CAD build for the part. Positions are in the model's coordinates, mm. A direction names the side the tool comes from. Round coordinates to 2 decimals unless told otherwise and drop trailing zeros. Write each loop counter-clockwise with the first axis right and the second up, starting at its lowest first coordinate (ties: lowest second). Pieces come first, ordered by that corner, then holes. Notation, with made-up numbers: M -39.75,-6.5 L -31.75,-6.5 A26 cw -31.75,29.5 Z; hole C 15,23 d2. An arc over 180 degrees is marked long. Write each question's results on one line, items separated by ' | '. Start each with the question number.
```python
from build123d import *

# Parameters (mm, degrees)
ESQUISSE1_R                        = 11
BOSS_EXTRU_1_DEPTH                 = 5
ESQUISSE2_R                        = 1
ENL_V_MAT_EXTRU_1_DEPTH            = 6
ESQUISSE3_R                        = 5
BOSS_EXTRU_2_DEPTH                 = 57.75
BOSS_EXTRU_3_DEPTH                 = 15
CONG_1_R                           = 1
R_P_TITION_CIRCULAIRE1_COUNT       = 5
CONG_1_OF_R_P_TITION_CIRCULAIRE1_R = 1


with BuildPart() as part:
    # Esquisse1 → Boss.-Extru.1 (new body)
    with BuildSketch(Plane.XY):
        Circle(ESQUISSE1_R)
    extrude(amount=BOSS_EXTRU_1_DEPTH)

    # Esquisse2 → Enlèv. mat.-Extru.1 (cut, through all)
    with BuildSketch(Plane.XY.offset(5)):
        with Locations((0, 8)):
            Circle(ESQUISSE2_R)
        with Locations((0, -8)):
            Circle(ESQUISSE2_R)
    extrude(amount=-ENL_V_MAT_EXTRU_1_DEPTH, mode=Mode.SUBTRACT)

    # Esquisse3 → Boss.-Extru.2 (add)
    with BuildSketch(Plane.XY.offset(5)):
        Circle(ESQUISSE3_R)
    extrude(amount=BOSS_EXTRU_2_DEPTH)

    # Esquisse4 → Boss.-Extru.3 (add, symmetric)
    with BuildSketch(Plane.XY.offset(35)):
        with BuildLine():
            ThreePointArc((-2.731158071, 4.188170912), (-2.5, 7.120566641), (-1.5, 9.886859967))
            ThreePointArc((-1.5, 9.886859967), (0, 10), (1.5, 9.886859967))
            ThreePointArc((1.5, 9.886859967), (2.5, 7.120566641), (2.731158071, 4.188170912))
            ThreePointArc((2.731158071, 4.188170912), (0, -5), (-2.731158071, 4.188170912))
        make_face()
    boss_extru_3 = extrude(amount=BOSS_EXTRU_3_DEPTH, both=True)

    # Congé1
    cong_1_edges = [part.edges().sort_by_distance(p)[0] for p in [
        (1.5, 9.886859967, 35),
        (-1.5, 9.886859967, 35),
    ]]
    fillet(cong_1_edges, radius=CONG_1_R)

    # Répétition circulaire1: Boss.-Extru.3 ×5 about axis
    r_p_tition_circulaire1_axis = Axis((0, 0, 0), (0, 0, 1))
    for i in range(1, R_P_TITION_CIRCULAIRE1_COUNT):
        add(boss_extru_3.rotate(r_p_tition_circulaire1_axis, i * 360 / R_P_TITION_CIRCULAIRE1_COUNT))

    # Congé1 of Répétition circulaire1
    cong_1_of_r_p_tition_circulaire1_edges = [part.edges().sort_by_distance(p)[0] for p in [
        (-8.939437105, 4.481792525, 35),
        (-9.866488089, 1.628622976, 35),
        (-7.024875971, -7.116959856, 35),
        (-4.597824988, -8.880315612, 35),
        (4.597824988, -8.880315612, 35),
        (7.024875971, -7.116959856, 35),
        (9.866488089, 1.628622976, 35),
        (8.939437105, 4.481792525, 35),
    ]]
    fillet(cong_1_of_r_p_tition_circulaire1_edges, radius=CONG_1_OF_R_P_TITION_CIRCULAIRE1_R)


solid = part.part
```
1) Saw through at A-A, the plane y = 8. Write the cut outline in (x, z).
2) Drop flat-ended pins along their axis: pin 1 Ø4 at (y, z) = (0, 43.5) entering from +X; pin 2 Ø12 at (x, z) = (-7.5, 36) entering from -Y; pin 3 Ø5 at (x, z) = (-1.5, 42.5) entering from +Y; pin 4 Ø1.8 at (x, y) = (0, -8) entering from -Z. Give the stop position or say it passes through.
3) 3-axis set-ups, long thin cutter, end or side, ignore diameter. For faces 4 (the face through (9.507, 3.103, 35.21)), 5 (the face through (4.77, 1.5, 14.22)), 6 (the face through (4, -6, 50)), 7 (the face through (-1.927, -7.013, 35.21)), 8 (the face through (0, 9, 3)): which of +Z, -Z, +X, -X, +Y, -Y reach the whole face in a straight line?
4) Wall check: line 1 along Y through (x, z) = (0, 2.95); line 2 along Z through (x, y) = (4.5, -5.5); line 3 along X through (y, z) = (-0.25, 19.5). Give the ranges that are in metal, low to high. Write a range as from..to.
5) Pull direction X, two halves, no side cores. Call faces 1 (the face through (-7, 2, 50)), 2 (the face through (5.68, 4.54, 35.21)), 3 (the face through (6.074, -3.999, 35.21)): pulls with the +X half, pulls with the -X half, needs draft (parallel to the pull), parting line crosses it, or undercut.
6) Saw through at B-B, the plane z = 11. Write the cut outline in (x, y), plus the area to 3 significant figures.
Filled sheet:
1) outline: M -7.55,0 L -1,0 L -1,5 L -7.55,5 Z; M -2.27,20 L 2.27,20 L 2.27,50 L -2.27,50 Z; M 1,0 L 7.55,0 L 7.55,5 L 1,5 Z
2) pin 1: stops at x = 9.78 | pin 2: stops at y = -8.74 | pin 3: stops at y = 10 | pin 4: passes through
3) face 4: +Z, +X, +Y | face 5: none | face 6: +Z, +X, -Y | face 7: +Z, -Y | face 8: -Z
4) line 1: y = -11..-9, -7..7, 9..11 | line 2: z = 0..5, 20..50 | line 3: x = -4.99..4.99
5) face 1: needs draft | face 2: undercut | face 3: pulls with the +X half
6) outline: C 0,0 d10 | area: 78.5 mm^2
